```python
from build123d import *

# Parameters (mm, degrees)
SKETCH_1_W          = 45
SKETCH_1_H          = 45
EXTRUDE_1_DEPTH     = 12
SKETCH_2_R          = 4
CUT_EXTRUDE_1_DEPTH = 5
SKETCH_3_R          = 4
CUT_EXTRUDE_2_DEPTH = 5
SKETCH_4_W          = 30
SKETCH_4_H          = 30
CUT_EXTRUDE_3_DEPTH = 2


with BuildPart() as part:
    # 草图1 → 凸台-拉伸1 (new body)
    with BuildSketch(Plane(origin=(0, 0, 0), x_dir=(1, 0, 0), z_dir=(0, 1, 0))):
        with Locations((22.5, 22.5)):
            Rectangle(SKETCH_1_W, SKETCH_1_H)
    extrude(amount=EXTRUDE_1_DEPTH)

    # 草图2 → 切除-拉伸1 (cut)
    with BuildSketch(Plane.XY):
        with Locations((22.5, 6)):
            Circle(SKETCH_2_R)
    extrude(amount=-CUT_EXTRUDE_1_DEPTH, mode=Mode.SUBTRACT)

    # 草图3 → 切除-拉伸2 (cut)
    with BuildSketch(Plane.ZY):
        with Locations((-22.477885381, 6)):
            Circle(SKETCH_3_R)
    extrude(amount=-CUT_EXTRUDE_2_DEPTH, mode=Mode.SUBTRACT)

    # 草图4 → 切除-拉伸3 (cut)
    with BuildSketch(Plane(origin=(0, 12, 0), x_dir=(1, 0, 0), z_dir=(0, 1, 0))):
        with Locations((22, 22)):
            Rectangle(SKETCH_4_W, SKETCH_4_H)
    extrude(amount=-CUT_EXTRUDE_3_DEPTH, mode=Mode.SUBTRACT)


solid = part.part
```
Read the model definition and answer for the solid it produces. Units are mm, in the model's axes. A direction names the side the tool comes from. Coordinates: 2 decimals unless noted, no trailing zeros. Write each loop counter-clockwise with the first axis right and the second up, starting at its lowest first coordinate (ties: lowest second). Pieces come first, ordered by that corner, then holes. Notation, with made-up numbers: (88.5, -3.75) -> (113.5, -3.75) arc R32 ccw to (113.5, 26.25) -> close; hole circle Ø5 at (18.25, -12). An arc over 180 degrees is marked (long way). Return JSON: item names as keys, results as strings.
1. A tool of negligible diameter and unlimited length cuts with its end or side. For faces 1 (the face through (19.3, 3.6, -2.5)), 2 (the face through (22, 11, -37)), 3 (the face through (2.46, 4.47, -18.78)), from which of +Z, -Z, +X, -X, +Y, -Y can it reach the whole face along a straight path? Write none if from no direction.
Found:
{"face 1": "+Z", "face 2": "+Y", "face 3": "-X"}
2. A cutting plane is placed at B-B (x = 12.5). Determine the outline of the cut face in (y, z).
Found:
{"outline": "(0, -45) -> (12, -45) -> (12, -37) -> (10, -37) -> (10, -7) -> (12, -7) -> (12, 0) -> (0, 0) -> close"}
3. A cutting plane is placed at D-D (y = 6). Determine the outline of the cut face in (x, z).
Found:
{"outline": "(0, -45) -> (45, -45) -> (45, 0) -> (26.5, 0) -> (26.5, -5) -> (18.5, -5) -> (18.5, 0) -> (0, 0) -> (0, -18.48) -> (5, -18.48) -> (5, -26.48) -> (0, -26.48) -> close"}
4. A cutting plane is placed at A-A (z = -15). Determine the outline of the cut face in (x, y), and give its area (3 significant figures).
Found:
{"outline": "(0, 0) -> (45, 0) -> (45, 12) -> (37, 12) -> (37, 10) -> (7, 10) -> (7, 12) -> (0, 12) -> close", "area": "480 mm2"}
5. Find the intervals of material crossed by line 1 along Y through (x, z) = (27, -20); line 2 along Z through (x, y) = (21, 8.75); line 3 along Y through (x, z) = (22.5, -2.3), in increasing order. Write a range as from..to.
Found:
{"line 1": "0..10", "line 2": "-45..-5", "line 3": "0..2, 10..12"}
6. Each of these flat-tipped pins is pushed along its axis until it touches: P1, Ø4, axis at x = 13.5, z = -28.5, coming from the -Y side; P2, Ø9, axis at x = 27.5, z = -22, coming from the +Y side; P3, Ø4, axis at x = 23.5, y = 6, coming from the +Z side. Where does it stop, or does it pass through?
Found:
{"P1": "y = 0", "P2": "y = 10", "P3": "z = -5"}
7. Determine the mould class of faces 4 (the face through (22, 11, -7)), 5 (the face through (22, 6, -45)), 6 (the face through (22, 12, -38)) for opening direction Z: pulls with the +Z half, pulls with the -Z half, needs draft (parallel to the pull), parting line crosses it, or undercut.
Found:
{"face 4": "undercut", "face 5": "pulls with the -Z half", "face 6": "needs draft"}
8. A cutting plane is placed at C-C (y = 10.75). Determine the outline of the cut face in (x, z).
Found:
{"outline": "(0, -45) -> (45, -45) -> (45, 0) -> (0, 0) -> close; hole (7, -37) -> (37, -37) -> (37, -7) -> (7, -7) -> close"}
